Could you check a few things on this model? Use its own coordinates, in mm. A direction names the side the tool comes from. Round coordinates to 2 decimals unless told otherwise and drop trailing zeros. Loops run counter-clockwise (first coordinate to the right, second up) from the corner with the lowest first, then second, coordinate; pieces in that order, holes last.
from build123d import *

# Parameters (mm, degrees)
CHAMFER_1_SIZE            = 1
CHAMFER_2_SIZE            = 0.5
SKETCH_2_W                = 2
SKETCH_2_H                = 25
CUT_EXTRUDE_695_DEPTH     = 50
HOLE_WIZARD_M3_1_D        = 3.4
HOLE_WIZARD_M3_1_2_REACH  = 111.075
HOLE_WIZARD_M3_1_2_BORE_R = 1.25


with BuildPart() as part:
    # 草图1 → 旋转1 (revolve)
    with BuildSketch(Plane.XY, mode=Mode.PRIVATE) as revolve_1_sk:
        Polygon((40, 0), (50, 0), (50, 4), (42.5, 4), (42.5, 48), (40, 48), align=None)
    revolve(revolve_1_sk.sketch.rotate(Axis((0, 0, 0), (0, 1, 0)), 90), axis=Axis((0, 0, 0), (0, 1, 0)))

    # 倒角1
    chamfer_1_edges = [part.edges().sort_by_distance(p)[0] for p in [
        (0, 4, 42.5),
    ]]
    chamfer(chamfer_1_edges, length=CHAMFER_1_SIZE)

    # 倒角2
    chamfer_2_edges = [part.edges().sort_by_distance(p)[0] for p in [
        (0, 48, 40),
    ]]
    chamfer(chamfer_2_edges, length=CHAMFER_2_SIZE)

    # 草图2 → Cut-Extrude 695 (cut, symmetric)
    with BuildSketch(Plane.XY):
        with Locations((0, 35.5)):
            Rectangle(SKETCH_2_W, SKETCH_2_H)
    extrude(amount=CUT_EXTRUDE_695_DEPTH, both=True, mode=Mode.SUBTRACT)

    # Hole Wizard M3 _1 (through all)
    with Locations(Plane(origin=(0, 0, 0), x_dir=(-1, 0, 0), z_dir=(0, -1, 0))):
        with Locations((0, 47), (40.703193978, 23.5), (40.703193978, -23.5), (0, -47), (-40.703193978, -23.5), (-40.703193978, 23.5)):
            Hole(HOLE_WIZARD_M3_1_D / 2)

    # Hole Wizard M3 _1 2 bore (on position points) → Hole Wizard M3 _1 2 (cut, up to next)
    with BuildSketch(Plane(origin=(42.5, 19, 0), x_dir=(0, 0, 1), z_dir=(1, 0, 0)), mode=Mode.PRIVATE) as hole_wizard_m3_1_2_sk1:
        Circle(HOLE_WIZARD_M3_1_2_BORE_R)
    hole_wizard_m3_1_2_tool1 = extrude(hole_wizard_m3_1_2_sk1.sketch, amount=-HOLE_WIZARD_M3_1_2_REACH, mode=Mode.PRIVATE) & part.part
    add(hole_wizard_m3_1_2_tool1.solids().sort_by_distance((42.5, 19, 0))[0], mode=Mode.SUBTRACT)


solid = part.part
Item 1: If we section it at B-B, the plane z = 0: Please give me the cut outline in (x, y).
Results list:
outline: (-50, 0) - (-40, 0) - (-40, 47.5) - (-40.5, 48) - (-42.5, 48) - (-42.5, 5) - (-43.5, 4) - (-50, 4) - close; (40, 0) - (50, 0) - (50, 4) - (43.5, 4) - (42.5, 5) - (42.5, 17.75) - (40, 17.75) - close; (40, 20.25) - (42.5, 20.25) - (42.5, 48) - (40.5, 48) - (40, 47.5) - close
Item 2: We'd pull the mould along Z, two halves only. Please class faces 1 (the cylindrical face through (-1.76, 23.42, 39.96)), 2 (the cylindrical face through (-12.766, 26.801, -40.537)), 3 (the flat face through (1, 35, -41)): released by +Z, released by -Z, zero draft, split by the parting line, or undercut.
Results list:
face 1: undercut
face 2: split by the parting line
face 3: zero draft
Item 3: If we section it at A-A, the plane y = 44.5: Please give me the cut outline in (x, z).
Results list:
outline: (-1, -42.49) - (-1, -39.99) arc R40 cw to (-1, 39.99) - (-1, 42.49) arc R42.5 ccw to start; (1, -42.49) arc R42.5 ccw to (1, 42.49) - (1, 39.99) arc R40 cw to (1, -39.99) - close
Item 4: If we section it at D-D, the plane y = 9.5: Please give me the cut outline in (x, z), then the cut area to 3 significant figures.
Results list:
outline: circle Ø85 at (0, 0); hole circle Ø80 at (0, 0)
area: 648 mm2
Item 5: Will these pins go through, and if not, where does the flat tip stop? pin 1 (6 mm diameter, centred on y = 32, z = 34, fed in from +X); pin 2 (8 mm diameter, centred on y = 26.5, z = -14.5, fed in from -X); pin 3 (6 mm diameter, centred on y = 33.5, z = 12.5, fed in from +X); pin 4 (2.5 mm diameter, centred on x = -40.7, z = 23.5, fed in from -Y) (3 decimals).
Results list:
pin 1: stops at x = 29.07
pin 2: stops at x = -41.18
pin 3: stops at x = 41.42
pin 4: passes through
Item 6: For faces 4 (the flat face through (-45, 4, 0)), 5 (the flat face through (1, 35, 41)), 6 (the flat face through (-34, 0, -22)), 7 (the cylindrical face through (40.482, 2.028, -25.186)), 8 (the cylindrical face through (41.26, 20.22, -0.27)), which set-ups out of +Z, -Z, +X, -X, +Y, -Y let a thin tool reach every point of the face, with its end or its side?
Results list:
face 4: +Y
face 5: +Z, -Z, +Y
face 6: +Z, -Z, +X, -X, -Y
face 7: +Y, -Y
face 8: +X
Item 7: If we section it at C-C, the plane z = -47: Please give me the cut outline in (x, y).
Results list:
outline: (-17.06, 0) - (-1.7, 0) - (-1.7, 4) - (-17.06, 4) - close; (1.7, 0) - (17.06, 0) - (17.06, 4) - (1.7, 4) - close
Item 8: If I drill on line 1 along X through (y, z) = (2, 23); line 2 along Z through (x, y) = (29, 28.5); line 3 along X through (y, z) = (31.5, -18), over which ranges is the centre line in solid material (lowest first)?
Results list:
line 1: x = -44.4 to -42.33, -39.08 to -32.73, 32.73 to 39.08, 42.33 to 44.4
line 2: z = -31.07 to -27.55, 27.55 to 31.07
line 3: x = -38.5 to -35.72, 35.72 to 38.5
